Verification items for this drawing (mm, ordinates from the low corner). A direction names the side the tool comes from. Coordinates: 2 decimals unless noted, no trailing zeros. Write each loop counter-clockwise with the first axis right and the second up, starting at its lowest first coordinate (ties: lowest second). Pieces come first, ordered by that corner, then holes. Notation, with made-up numbers: (15.25, 74.25) -> (45.25, 74.25) arc R14 cw to (45.25, 90.25) -> close; hole circle Ø5 at (46, 48). An arc over 180 degrees is marked (long way). Use CSV: the item, a comma, the result in double quotes.
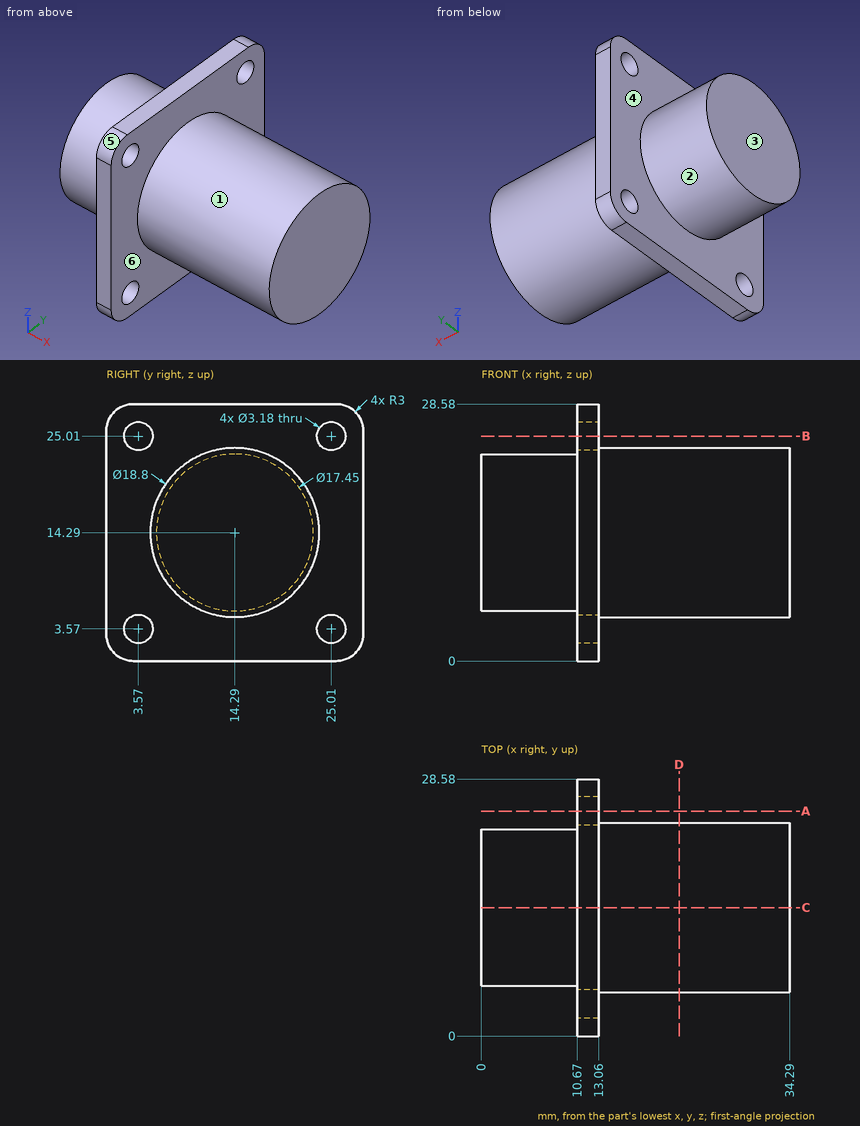
1) Cross-section at D-D (x = 22). Record the boundary of the cut face in (y, z), plus the area to 3 significant figures.
Return value:
outline,"circle Ø18.8 at (14.29, 14.29)"
area,"278 mm2"
2) Set-up check for the marked faces 1, 2 and 3: record each of +Z, -Z, +X, -X, +Y, -Y from which the full face is reachable in a straight line by a thin tool's end or side.
Return value:
face 1,"+X"
face 2,"-X"
face 3,"+Z, -Z, -X, +Y, -Y"
3) Cross-section at C-C (y = 14.29). Record the boundary of the cut face in (x, z) (3 decimals).
Return value:
outline,"(0, 5.565) -> (10.67, 5.565) -> (10.67, 0) -> (13.06, 0) -> (13.06, 4.89) -> (34.29, 4.89) -> (34.29, 23.69) -> (13.06, 23.69) -> (13.06, 28.58) -> (10.67, 28.58) -> (10.67, 23.015) -> (0, 23.015) -> close"
4) Mould release check, pull along X, two halves, no side actions. Record for the marked faces 4, 5 and 6: released by +X, released by -X, zero draft, split by the parting line, or undercut.
Return value:
face 4,"released by -X"
face 5,"zero draft"
face 6,"released by +X"
5) Scan lines: L1, parallel to Y at x = 12.5, z = 25.01; L2, parallel to Y at x = 13, z = 4.5; L3, parallel to X at y = 23.5, z = 10.25. Record each from-to range of solid material in increasing order.
Return value:
L1,"0 to 1.98, 5.16 to 23.42, 26.6 to 28.58"
L2,"0 to 2.28, 4.86 to 23.72, 26.3 to 28.58"
L3,"10.67 to 13.06"
6) Gauge pin test, flat ends, axial feed: pin 1 (4 mm diameter, centred on y = 25.01, z = 25.01, fed in from -X); pin 2 (3 mm diameter, centred on x = 15.5, y = 14.5, fed in from -Z); pin 3 (3.5 mm diameter, centred on y = 3.57, z = 3.57, fed in from +X). Record the tip position at first contact, or that the pin passes through.
Return value:
pin 1,"x = 10.67"
pin 2,"z = 4.89"
pin 3,"x = 13.06"
7) Cross-section at A-A (y = 25.01). Record the boundary of the cut face in (x, z), plus the area to 3 significant figures.
Return value:
outline,"(10.67, 0) -> (13.06, 0) -> (13.06, 1.98) -> (10.67, 1.98) -> close; (10.67, 5.16) -> (13.06, 5.16) -> (13.06, 23.42) -> (10.67, 23.42) -> close; (10.67, 26.6) -> (13.06, 26.6) -> (13.06, 28.58) -> (10.67, 28.58) -> close"
area,"53.1 mm2"
